Model file for the job. Use its own axes, mm. A direction names the side the tool comes from. Give positions to 0.01 mm unless a question says otherwise; leave off trailing zeros. Write each loop counter-clockwise with the first axis right and the second up, starting at its lowest first coordinate (ties: lowest second). Pieces come first, ordered by that corner, then holes.
```python
from build123d import *

# Parameters (mm, degrees)
SKETCH_R           = 0.65
PAD_DEPTH          = 5
SKETCH001_W        = 19.2
SKETCH001_H        = 6.5
SKETCH001_W_2      = 15.2
SKETCH001_H_2      = 2.5
SKETCH001_W_3      = 6.5
SKETCH001_H_3      = 19.2
SKETCH001_W_4      = 2.5
SKETCH001_H_4      = 15.2
PAD001_DEPTH       = 5
POLARPATTERN_COUNT = 4
SKETCH002_W        = 88.84
SKETCH002_H        = 88.84
POCKET_DEPTH       = 5.001
SKETCH003_W        = 135.310039
SKETCH003_H        = 121.25861
SKETCH003_W_2      = 101.84
SKETCH003_H_2      = 101.84
POCKET001_DEPTH    = 4.9


with BuildPart() as part:
    # Sketch → Pad (new body)
    with BuildSketch(Plane.XY):
        Polygon((-52.00016, -52.00016), (0, -52.00016), (0, -42.00016), (-34.929092, -42.00016), (0, -7.071068), (0, 0), (-7.071068, 0), (-42.00016, -34.929092), (-42.00016, 0), (-52.00016, 0), align=None)
        with Locations((-47.00016, -47.00016)):
            Circle(SKETCH_R, mode=Mode.SUBTRACT)
        with Locations((-26.67, -26.67)):
            Circle(SKETCH_R, mode=Mode.SUBTRACT)
    pad = extrude(amount=PAD_DEPTH)

    # Sketch001 (on Face14 of Pad) → Pad001 (join)
    with BuildSketch(Plane.XY.offset(5)):
        with Locations((-26.67, -47.67)):
            Rectangle(SKETCH001_W, SKETCH001_H)
        with Locations((-26.67, -47.67)):
            Rectangle(SKETCH001_W_2, SKETCH001_H_2, mode=Mode.SUBTRACT)
        with Locations((-47.67, -26.67)):
            Rectangle(SKETCH001_W_3, SKETCH001_H_3)
        with Locations((-47.67, -26.67)):
            Rectangle(SKETCH001_W_4, SKETCH001_H_4, mode=Mode.SUBTRACT)
    pad001 = extrude(amount=PAD001_DEPTH)

    # PolarPattern: Pad, Pad001 ×4 about axis
    polarpattern_axis = Axis((0, 0, 0), (0, 0, 1))
    for i in range(1, POLARPATTERN_COUNT):
        add(pad.rotate(polarpattern_axis, i * 360 / POLARPATTERN_COUNT))
        add(pad001.rotate(polarpattern_axis, i * 360 / POLARPATTERN_COUNT))

    # Sketch002 (on Face20 of PolarPattern) → Pocket (cut, through all)
    with BuildSketch(Plane.XY.offset(5)):
        Rectangle(SKETCH002_W, SKETCH002_H)
    extrude(amount=-POCKET_DEPTH, mode=Mode.SUBTRACT)

    # Sketch003 (on Face5 of Pocket) → Pocket001 (cut)
    with BuildSketch(Plane.XY.offset(5)):
        with Locations((8.080424, -2.412195)):
            Rectangle(SKETCH003_W, SKETCH003_H)
        Rectangle(SKETCH003_W_2, SKETCH003_H_2, mode=Mode.SUBTRACT)
    extrude(amount=-POCKET001_DEPTH, mode=Mode.SUBTRACT)


solid = part.part
```
1. Slice it at C-C, the plane y = -29. Write the cut outline in (x, z), and give its area (3 significant figures).
Calculated:
outline: (-52, 0) - (-44.42, 0) - (-44.42, 10) - (-46.42, 10) - (-46.42, 5) - (-48.92, 5) - (-48.92, 10) - (-50.92, 10) - (-50.92, 0.1) - (-52, 0.1) - close; (44.42, 0) - (52, 0) - (52, 0.1) - (50.92, 0.1) - (50.92, 10) - (48.92, 10) - (48.92, 5) - (46.42, 5) - (46.42, 10) - (44.42, 10) - close
area: 105 mm2
2. Probe probe 1 along X at (y, z) = (-47, 9); probe 2 along X at (y, z) = (32, 8.5); probe 3 along Y at (x, z) = (38.5, 3). List the from-to ranges inside material, lowest first.
Calculated:
probe 1: x = -36.27 to -34.27, -19.07 to -17.07, 17.07 to 19.07, 34.27 to 36.27
probe 2: x = -50.92 to -48.92, -46.42 to -44.42, 44.42 to 46.42, 48.92 to 50.92
probe 3: y = -50.92 to -44.42, 44.42 to 50.92
3. Which spindle directions (+Z, -Z, +X, -X, +Y, -Y) get a long thin tool onto all of the face, cutting with end or side? Do faces 1 (the flat face through (-17.07, -48, 7)), 2 (the flat face through (-27, 46.42, 7)), 3 (the flat face through (-1, -44.42, 4)). Say none if no direction does.
Calculated:
face 1: +Z, +Y, -Y
face 2: +Z
face 3: +Z, -Z
4. Pull direction X, two halves, no side cores. Call faces 4 (the flat face through (27, 48, 5)), 5 (the flat face through (48, 36.27, 7)): +X half, -X half, draft (parallel to the pull), parting line (faces both ways), or undercut.
Calculated:
face 4: undercut
face 5: draft
5. Slice it at D-D, the plane z = 7.5. State how many separate pieces and enclosed holes the cut face has, and give its area (3 significant figures).
Calculated:
separate pieces: 8
enclosed holes: 8
area: 694 mm2
6. Pin check, flat tips, straight feed: P1, Ø4, axis at y = -24.5, z = 6.5, coming from the -X side; P2, Ø5, axis at x = -34.5, z = 4.5, coming from the +Y side; P3, Ø6, axis at y = 6, z = 5.5, coming from the +X side; P4, Ø1.5, axis at x = 3.5, z = 7, coming from the +Y side. Stop position of each tip, or through.
Calculated:
P1: stops at x = -50.92
P2: stops at y = 50.92
P3: stops at x = 50.92
P4: passes through
7. Slice it at A-A, the plane x = -3.5. Write the cut outline in (y, z).
Calculated:
outline: (-52, 0) - (-44.42, 0) - (-44.42, 5) - (-50.92, 5) - (-50.92, 0.1) - (-52, 0.1) - close; (44.42, 0) - (52, 0) - (52, 0.1) - (50.92, 0.1) - (50.92, 5) - (44.42, 5) - close
